The model under review builds one solid part; all positions refer to its coordinate system, in mm. Give positions to 0.01 mm unless a question says otherwise; leave off trailing zeros. Loops run counter-clockwise (first coordinate to the right, second up) from the corner with the lowest first, then second, coordinate; pieces in that order, holes last. Notation, with made-up numbers: M -4.5,13 L 25.5,13 A31 ccw 25.5,44 Z; hole C 29.5,-4 d10. An arc over 180 degrees is marked long. Write item = value, one per line. Start each with the question number.
1. We need section A-A on x = 18.5. Give the boundary of the cut face in (y, z).
2. For pin 1 (1.6 mm diameter, centred on y = 3.5, z = 18, fed in from +X); pin 2 (1 mm diameter, centred on x = 12.5, y = 3, fed in from -Z); pin 3 (4 mm diameter, centred on x = 40, z = -99.5, fed in from +Y); pin 4 (2.5 mm diameter, centred on x = -40, z = -99.5, fed in from -Y), all flat-tipped, find the tip position at first contact; note any pin that passes through.
3. Wall thickness on line 1 along X through (y, z) = (0.95, -99.5); line 2 along X through (y, z) = (0.7, -99.5); line 3 along Z through (x, y) = (-17, 2.75): over which ranges is each line inside the solid? List them lowest first. Write a range as from..to.
4. We need section B-B on z = -10. Give the boundary of the cut face in (x, y).
from build123d import *

# Parameters (mm, degrees)
SKETCH1_W                 = 88
SKETCH1_H                 = 207
BOSS_EXTRUDE1_DEPTH       = 2
SKETCH2_W                 = 78
SKETCH2_H                 = 199
BOSS_EXTRUDE2_DEPTH       = 2
CHAMFER1_SIZE             = 5
FILLET1_R                 = 5
F_3_0MM_DOWEL_HOLE1_D     = 3
F_3_0MM_DOWEL_HOLE1_DEPTH = 17.29
F_3_0MM_DOWEL_HOLE1_TIP   = 0.901290929
CHAMFER2_SIZE             = 1


with BuildPart() as part:
    # Sketch1 → Boss-Extrude1 (new body)
    with BuildSketch(Plane(origin=(0, 0, 0), x_dir=(1, 0, 0), z_dir=(0, 1, 0))):
        Rectangle(SKETCH1_W, SKETCH1_H)
    extrude(amount=BOSS_EXTRUDE1_DEPTH)

    # Sketch2 → Boss-Extrude2 (add)
    with BuildSketch(Plane(origin=(0, 2, 0), x_dir=(1, 0, 0), z_dir=(0, 1, 0))):
        Rectangle(SKETCH2_W, SKETCH2_H)
    extrude(amount=BOSS_EXTRUDE2_DEPTH)

    # Chamfer1
    chamfer1_edges = [part.edges().sort_by_distance(p)[0] for p in [
        (39, 3, 99.5),
        (39, 3, -99.5),
        (-39, 3, -99.5),
        (-39, 3, 99.5),
    ]]
    chamfer(chamfer1_edges, length=CHAMFER1_SIZE)

    # Fillet1
    fillet1_edges = [part.edges().sort_by_distance(p)[0] for p in [
        (-39, 3, 94.5),
        (-39, 3, -94.5),
        (34, 3, -99.5),
        (-34, 3, -99.5),
        (39, 3, 94.5),
        (39, 3, -94.5),
        (34, 3, 99.5),
        (-34, 3, 99.5),
        (44, 1, 103.5),
        (-44, 1, 103.5),
        (-44, 1, -103.5),
        (44, 1, -103.5),
    ]]
    fillet(fillet1_edges, radius=FILLET1_R)

    # Ø3.0mm Dowel Hole1
    with Locations(Plane(origin=(0, 0, 0), x_dir=(-1, 0, 0), z_dir=(0, -1, 0))):
        with Locations((-40, 99.5), (40, 99.5), (40, -99.5), (-40, -99.5)):
            Hole(F_3_0MM_DOWEL_HOLE1_D / 2, depth=F_3_0MM_DOWEL_HOLE1_DEPTH)
            with Locations((0, 0, -(F_3_0MM_DOWEL_HOLE1_DEPTH + F_3_0MM_DOWEL_HOLE1_TIP / 2))):  # 118° drill point
                Cone(0, F_3_0MM_DOWEL_HOLE1_D / 2, F_3_0MM_DOWEL_HOLE1_TIP, mode=Mode.SUBTRACT)

    # Chamfer2
    chamfer2_edges = [part.edges().sort_by_distance(p)[0] for p in [
        (0, 0, 103.5),
        (44, 0, 0),
        (-44, 0, 0),
        (0, 0, -103.5),
        (-42.535533906, 0, -102.035533906),
        (42.535533906, 0, -102.035533906),
        (42.535533906, 0, 102.035533906),
        (-42.535533906, 0, 102.035533906),
    ]]
    chamfer(chamfer2_edges, length=CHAMFER2_SIZE)


solid = part.part
Final values:
q1.outline = M 0,-102.5 L 1,-103.5 L 2,-103.5 L 2,-99.5 L 4,-99.5 L 4,99.5 L 2,99.5 L 2,103.5 L 1,103.5 L 0,102.5 Z
q2.pin_1 = 39
q2.pin_2 = -99.5
q2.pin_3 = 2
q2.pin_4 = through
q3.line_1 = -43.85..-41.5, -38.5..38.5, 41.5..43.85
q3.line_2 = -43.59..-41.5, -38.5..38.5, 41.5..43.59
q3.line_3 = -99.5..99.5
q4.outline = M -44,1 L -43,0 L 43,0 L 44,1 L 44,2 L 39,2 L 39,4 L -39,4 L -39,2 L -44,2 Z
